Part model, mm, in its own coordinate system. Give positions to 0.01 mm unless a question says otherwise; leave off trailing zeros. Order: outer loops, then holes, each group sorted by start corner. A loop starts at its lowest first (then second) coordinate and runs counter-clockwise, first axis right, second up. Notation, with made-up numbers: M -35,32.25 L -10,32.25 A13 cw -10,40.25 Z; hole C -11,42.5 d4. An arc over 180 degrees is marked long. Return JSON: item names as keys, results as strings.
from build123d import *

# Parameters (mm, degrees)
SKETCH1_R           = 11.7094
SKETCH1_R_2         = 10.4648
BOSS_EXTRUDE1_DEPTH = 2501.9
SKETCH2_R           = 3.3782
CUT_EXTRUDE1_DEPTH  = 12.7094


with BuildPart() as part:
    # Sketch1 → Boss-Extrude1 (new body)
    with BuildSketch(Plane(origin=(0, 0, 0), x_dir=(0, 0, -1), z_dir=(1, 0, 0))):
        Circle(SKETCH1_R)
        Circle(SKETCH1_R_2, mode=Mode.SUBTRACT)
    extrude(amount=BOSS_EXTRUDE1_DEPTH)

    # Sketch2 → Cut-Extrude1 (cut, symmetric)
    with BuildSketch(Plane(origin=(0, 0, 0), x_dir=(1, 0, 0), z_dir=(0, 1, 0))):
        with Locations((12.7, 0)):
            Circle(SKETCH2_R)
    cut_extrude1 = extrude(amount=CUT_EXTRUDE1_DEPTH, both=True, mode=Mode.SUBTRACT)

    # Mirror1: Cut-Extrude1 across plane
    add(cut_extrude1.mirror(Plane.ZY.offset(-1250.95)), mode=Mode.SUBTRACT)


solid = part.part
Q1. Probe line 1 along X through (y, z) = (10.9, 0); line 2 along Y through (x, z) = (862, 0); line 3 along Z through (x, y) = (1075, 3.25). List the from-to ranges inside material, lowest first.
Established:
{"line 1": "x = 0 to 9.32, 16.08 to 2485.82, 2492.58 to 2501.9", "line 2": "y = -11.71 to -10.46, 10.46 to 11.71", "line 3": "z = -11.25 to -9.95, 9.95 to 11.25"}
Q2. Band-saw the part on A-A (y = 0). Give the cut face in (x, z), then the cut area to 3 significant figures.
Established:
{"outline": "M 0,-11.71 L 2501.9,-11.71 L 2501.9,-10.46 L 0,-10.46 Z; M 0,10.46 L 2501.9,10.46 L 2501.9,11.71 L 0,11.71 Z", "area": "6,230 mm²"}
Q3. Band-saw the part on B-B (x = 1548). Give the cut face in (y, z), then the cut area to 3 significant figures.
Established:
{"outline": "C 0,0 d23.42; hole C 0,0 d20.93", "area": "86.7 mm²"}
Q4. Pin check, flat tips, straight feed: pin 1 (12 mm diameter, centred on y = -1, z = -1, fed in from +X); pin 2 (1 mm diameter, centred on x = 1840, y = -2, fed in from +Z); pin 3 (8 mm diameter, centred on x = 901.5, z = -4.5, fed in from -Y); pin 4 (1 mm diameter, centred on x = 795, z = -5, fed in from +Y). Stop position of each tip, or through.
Established:
{"pin 1": "passes through", "pin 2": "stops at z = 11.61", "pin 3": "stops at y = -11.7", "pin 4": "stops at y = 10.81"}
